```python
from build123d import *

# Parameters (mm, degrees)
ESBO_O1_R                = 7.44
ESBO_O1_R_2              = 6.6
RESSALTO_EXTRUS_O1_DEPTH = 3.25
ESBO_O2_R                = 8.5
RESSALTO_EXTRUS_O2_DEPTH = 0.6
ESBO_O3_R                = 6.6
CORTE_EXTRUS_O1_DEPTH    = 15.275503494


with BuildPart() as part:
    # Esboço1 → Ressalto-extrusão1 (new, symmetric)
    with BuildSketch(Plane(origin=(0, 0, 0), x_dir=(0, 0, -1), z_dir=(1, 0, 0))):
        with Locations(Location((0, 0, 0), (0, 0, 180))):
            Circle(ESBO_O1_R)
        with Locations(Location((0, 0, 0), (0, 0, 180))):
            Circle(ESBO_O1_R_2, mode=Mode.SUBTRACT)
    extrude(amount=RESSALTO_EXTRUS_O1_DEPTH, both=True)

    # Esboço2 → Ressalto-extrusão2 (add)
    with BuildSketch(Plane(origin=(3.25, 0, 0), x_dir=(0, 0, -1), z_dir=(1, 0, 0))):
        Circle(ESBO_O2_R)
    ressalto_extrus_o2 = extrude(amount=RESSALTO_EXTRUS_O2_DEPTH)

    # Espelhar1: Ressalto-extrusão2 across plane
    add(ressalto_extrus_o2.mirror(Plane(origin=(0, 0, 0), x_dir=(0, 0, 1), z_dir=(1, 0, 0))))

    # Esboço3 → Corte-extrusão1 (cut, through all)
    with BuildSketch(Plane(origin=(3.85, 0, 0), x_dir=(0, 0, -1), z_dir=(1, 0, 0))):
        with Locations(Location((0, 0, 0), (0, 0, 180))):
            Circle(ESBO_O3_R)
    extrude(amount=-CORTE_EXTRUS_O1_DEPTH, mode=Mode.SUBTRACT)


solid = part.part
```
Geometry check sheet. Reference: the model listing, model coordinates, mm. A direction names the side the tool comes from. Coordinates: 2 decimals unless noted, no trailing zeros. Loops run counter-clockwise (first coordinate to the right, second up) from the corner with the lowest first, then second, coordinate; pieces in that order, holes last.
Item 1: Access from +Z, -Z, +X, -X, +Y, -Y to the whole of each face (thin tool, end or side, straight path). Record for faces 1 (the face through (0.046, -0.327, -7.433)), 2 (the face through (3.546, 7.167, -4.57)).
Item 2: Sectioned sample at C-C, the plane x = -2.5. Record the boundary of the cut face in (y, z).
Item 3: Thickness scan on line 1 (Y direction, x = 2, z = 0); line 2 (X direction, y = -6.5, z = 3.75). Record the ranges inside material, lowest first.
Item 4: Release check for a two-part mould opening along X. For faces 3 (the face through (3.85, -6.3, -2.5)), 4 (the face through (-3.85, -6.3, -2.5)), 5 (the face through (-3.25, -8, 0)) record: released by +X, released by -X, zero draft, split by the parting line, or undercut.
Item 5: Go/stop test with flat-tipped pins: pin 1 Ø4 at (x, y) = (0.5, 2) entering from +Z; pin 2 Ø8 at (y, z) = (0, 0) entering from +X; pin 3 Ø1.5 at (x, z) = (-1.5, -3.5) entering from -Y; pin 4 Ø1 at (y, z) = (-1, -6.5) entering from +X. Record where each tip stops, or that it passes through.
Item 6: Sectioned sample at A-A, the plane y = 0. Record the boundary of the cut face in (x, z).
Check result:
1. face 1: none
1. face 2: +X, -X
2. outline: circle Ø14.88 at (0, 0); hole circle Ø13.2 at (0, 0)
3. line 1: y = -7.44 to -6.6, 6.6 to 7.44
3. line 2: x = -3.85 to -3.25, 3.25 to 3.85
4. face 3: released by +X
4. face 4: released by -X
4. face 5: undercut
5. pin 1: stops at z = 7.44
5. pin 2: passes through
5. pin 3: stops at y = -6.91
5. pin 4: stops at x = 3.85
6. outline: (-3.85, -8.5) - (-3.25, -8.5) - (-3.25, -7.44) - (3.25, -7.44) - (3.25, -8.5) - (3.85, -8.5) - (3.85, -6.6) - (-3.85, -6.6) - close; (-3.85, 6.6) - (3.85, 6.6) - (3.85, 8.5) - (3.25, 8.5) - (3.25, 7.44) - (-3.25, 7.44) - (-3.25, 8.5) - (-3.85, 8.5) - close
